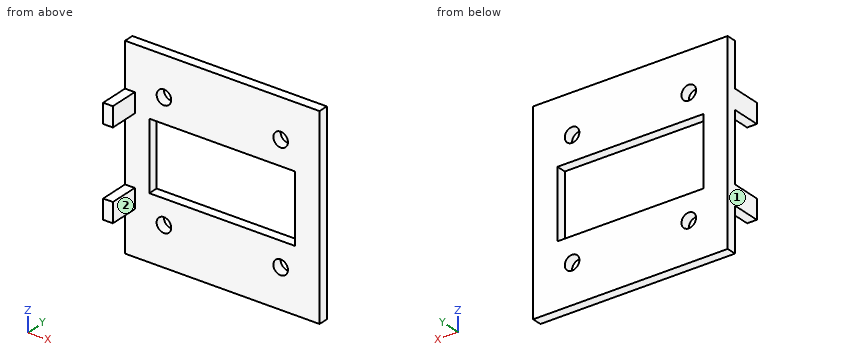
from build123d import *

# Parameters (mm, degrees)
SKETCH2_W           = 40
SKETCH2_H           = 40
SKETCH2_R           = 1.5
SKETCH2_W_2         = 30
SKETCH2_H_2         = 14.001199324
BOSS_EXTRUDE1_DEPTH = 2
SKETCH3_W           = 2
SKETCH3_H           = 4
BOSS_EXTRUDE2_DEPTH = 6


with BuildPart() as part:
    # Sketch2 → Boss-Extrude1 (new body)
    with BuildSketch(Plane(origin=(0, 0, 0), x_dir=(1, 0, 0), z_dir=(0, 1, 0))):
        Rectangle(SKETCH2_W, SKETCH2_H)
        with Locations(Location((-12, 12, 0), (0, 0, 270))):
            Circle(SKETCH2_R, mode=Mode.SUBTRACT)
        with Locations(Location((12, 12, 0), (0, 0, 270))):
            Circle(SKETCH2_R, mode=Mode.SUBTRACT)
        with Locations(Location((-12, -12, 0), (0, 0, 270))):
            Circle(SKETCH2_R, mode=Mode.SUBTRACT)
        with Locations(Location((12, -12, 0), (0, 0, 270))):
            Circle(SKETCH2_R, mode=Mode.SUBTRACT)
        Rectangle(SKETCH2_W_2, SKETCH2_H_2, mode=Mode.SUBTRACT)
    extrude(amount=BOSS_EXTRUDE1_DEPTH)

    # Sketch3 → Boss-Extrude2 (add)
    with BuildSketch(Plane.XZ):
        with Locations((-19, 9)):
            Rectangle(SKETCH3_W, SKETCH3_H)
        with Locations((-19, -9)):
            Rectangle(SKETCH3_W, SKETCH3_H)
    extrude(amount=BOSS_EXTRUDE2_DEPTH)


solid = part.part
Input: part model. Units: mm. Frame: model coordinates. Face numbers are marked on the shaded views. A direction names the side the tool comes from. Round coordinates to 2 decimals unless told otherwise and drop trailing zeros. Order: outer loops, then holes, each group sorted by start corner. A loop starts at its lowest first (then second) coordinate and runs counter-clockwise, first axis right, second up.
1. Cut plane A-A, the plane x = 12. Output: boundary loops of the cut face in (y, z).
The answers:
outline: (0, -20) - (2, -20) - (2, -13.5) - (0, -13.5) - close; (0, -10.5) - (2, -10.5) - (2, -7) - (0, -7) - close; (0, 7) - (2, 7) - (2, 10.5) - (0, 10.5) - close; (0, 13.5) - (2, 13.5) - (2, 20) - (0, 20) - close
2. Cut plane C-C, the plane x = -9. Output: boundary loops of the cut face in (y, z).
The answers:
outline: (0, -20) - (2, -20) - (2, -7) - (0, -7) - close; (0, 7) - (2, 7) - (2, 20) - (0, 20) - close
3. Pin query (flat end, axial travel): P1, Ø1.5, axis at x = -12, z = 6, coming from the +Y side; P2, Ø2, axis at x = -19, y = -3, coming from the -Z side; P3, Ø1, axis at x = -19, y = -4, coming from the +Z side; P4, Ø5, axis at x = 12, z = -12, coming from the -Y side. Return the tip coordinate at first contact, or that it passes through.
The answers:
P1: passes through
P2: stops at z = -11
P3: stops at z = 11
P4: stops at y = 0
4. Cut plane D-D, the plane z = 12. Output: boundary loops of the cut face in (x, y).
The answers:
outline: (-20, 0) - (-13.5, 0) - (-13.5, 2) - (-20, 2) - close; (-10.5, 0) - (10.5, 0) - (10.5, 2) - (-10.5, 2) - close; (13.5, 0) - (20, 0) - (20, 2) - (13.5, 2) - close
5. Cut plane B-B, the plane y = -3.5. Output: boundary loops of the cut face in (x, z).
The answers:
outline: (-20, -11) - (-18, -11) - (-18, -7) - (-20, -7) - close; (-20, 7) - (-18, 7) - (-18, 11) - (-20, 11) - close
6. Set-up query: the marked faces 1 and 2. Return all of +Z, -Z, +X, -X, +Y, -Y with unobstructed straight access to the full face (end or side cutting, diameter ignored); none if empty.
The answers:
face 1: +Z, -Z, -X, +Y, -Y
face 2: +Z, -Z, +X, -Y
7. Material intervals for line 1 (X direction, y = 1, z = -12); line 2 (Z direction, x = 0, y = 1.25); line 3 (Z direction, x = -11, y = 0.5), sorted ascending.
The answers:
line 1: x = -20 to -13.5, -10.5 to 10.5, 13.5 to 20
line 2: z = -20 to -7, 7 to 20
line 3: z = -20 to -13.12, -10.88 to -7, 7 to 10.88, 13.12 to 20
